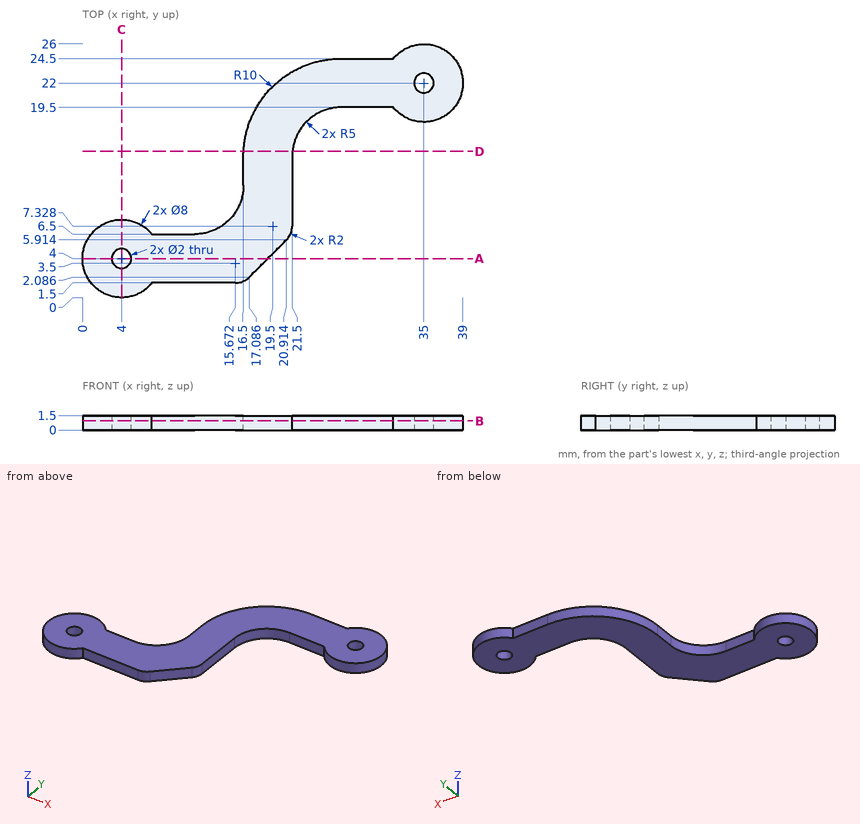
Here's the drawing with two shaded views (mm, measured from the low corner). I have some questions. Round coordinates to 2 decimals unless told otherwise and drop trailing zeros. Loops run counter-clockwise (first coordinate to the right, second up) from the corner with the lowest first, then second, coordinate; pieces in that order, holes last.
Item 1: Suppose I cut it at C-C, the plane x = 4. Write out the boundary of the cut face in (y, z).
Item 2: Suppose I cut it at B-B, the plane z = 0.95. Write out the boundary of the cut face in (x, y) (1 decimal).
Item 3: Suppose I cut it at D-D, the plane y = 15. Write out the boundary of the cut face in (x, z) (1 decimal).
Item 4: Please list where these lines run through material, in increasing order: L1, parallel to Y at x = 4, z = 0.4; L2, parallel to Y at x = 30.5, z = 0.2; L3, parallel to Y at x = 35, z = 0.7.
Item 5: Will this pin go through, and if not, where does the flat tip stop? pin 1 Ø1.2 at (x, y) = (35, 22) entering from +Z.
Item 6: Suppose I cut it at A-A, the plane y = 4. Write out the boundary of the cut face in (x, z), then the cut area to 3 significant figures.
Reported:
1. outline: (0, 0) - (3, 0) - (3, 1.5) - (0, 1.5) - close; (5, 0) - (8, 0) - (8, 1.5) - (5, 1.5) - close
2. outline: (7.1, 1.5) - (15.7, 1.5) arc R2 ccw to (17.1, 2.1) - (20.9, 5.9) arc R2 ccw to (21.5, 7.3) - (21.5, 14.5) arc R5 cw to (26.5, 19.5) - (31.9, 19.5) arc R4 ccw (long way) to (31.9, 24.5) - (26.5, 24.5) arc R10 ccw to (16.5, 14.5) - (16.5, 11.5) arc R5 cw to (11.5, 6.5) - (7.1, 6.5) arc R4 ccw (long way) to start; hole circle Ø2 at (4, 4); hole circle Ø2 at (35, 22)
3. outline: (16.5, 0) - (21.5, 0) - (21.5, 1.5) - (16.5, 1.5) - close
4. L1: y = 0 to 3, 5 to 8
4. L2: y = 19.5 to 24.5
4. L3: y = 18 to 21, 23 to 26
5. pin 1: passes through
6. outline: (0, 0) - (3, 0) - (3, 1.5) - (0, 1.5) - close; (5, 0) - (19, 0) - (19, 1.5) - (5, 1.5) - close
6. area: 25.5 mm2
